Can you work these out from the model? Positions are in its coordinate system, mm. Round coordinates to 2 decimals unless told otherwise and drop trailing zeros. Write each loop counter-clockwise with the first axis right and the second up, starting at its lowest first coordinate (ties: lowest second). Pieces come first, ordered by that corner, then holes. Notation, with made-up numbers: M -19,19 L 37,19 A21 cw 37,40 Z; hole C 63.5,78.5 d3. An arc over 180 degrees is marked long. Use one line per item in the form item = value. Start each with the question number.
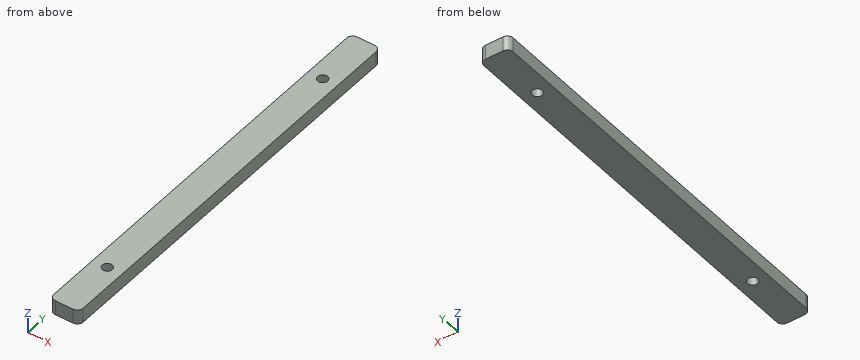
Autodesk Inventor part; units mm, degrees
ref_plane "YZ Plane" through (0, 0, 0) normal (1, 0, 0) x (0, 1, 0)
ref_plane "XZ Plane" through (0, 0, 0) normal (0, 1, 0) x (-1, 0, 0)
ref_plane "XY Plane" through (0, 0, 0) normal (0, 0, 1) x (1, 0, 0)
sketch "Sketch1" plane through (0, 0, 0) normal (0, 0, 1) x (1, 0, 0)
  line L0 (-5, -70) -> (5, -70)
  line L1 (5, -70) -> (5, 70)
  line L2 (5, 70) -> (-5, 70)
  line L3 (-5, 70) -> (-5, -70)
  line L4 (-5, -70) -> (5, 70) construction
  line L5 (5, -70) -> (-5, 70) construction
  point P0 (0, 0)
  dimension "d0" = 10
  dimension "d1" = 140
extrude "Extrusion1" add sketch "Sketch1" along normal blind 5
sketch "Sketch2" plane through (0, 0, 5) normal (0, 0, 1) x (1, 0, 0)
  line L0 (0, 50) -> (0, -50) construction
  point P0 (0, 0)
  point P1 (0, 0)
  dimension "d4" = 100
hole "Hole1" at (0, 50, 5) at (0, -50, 5) direction (0, 0, -1) diameter 3.4 depth 8 tip angle 118
fillet "Fillet1" radius 2 4 edges at (5, 70, 2.5) (-5, 70, 2.5) (5, -70, 2.5) (-5, -70, 2.5)
properties part number "ToslinkHalter" material "Polycarbonate, Clear"
1. If we section it at B-B (x = 0): List the corners of the cut face in (y, z) for me.
2. Will this pin go through, and if not, where does the flat tip stop? pin 1 (4 mm diameter, centred on x = 3.5, y = -12.5, fed in from -Z).
3. If we section it at A-A (y = -50): List the corners of the cut face in (x, z) for me, and give its area (3 significant figures).
4. Please list where these lines run through material, in increasing order: line 1 along Y through (x, z) = (0, 1.4); line 2 along X through (y, z) = (50, 3.45); line 3 along Y through (x, z) = (1, 0.3).
Model answer:
q1.outline = M -70,0 L -51.7,0 L -51.7,5 L -70,5 Z; M -48.3,0 L 48.3,0 L 48.3,5 L -48.3,5 Z; M 51.7,0 L 70,0 L 70,5 L 51.7,5 Z
q2.pin_1 = 0
q3.outline = M -5,0 L -1.7,0 L -1.7,5 L -5,5 Z; M 1.7,0 L 5,0 L 5,5 L 1.7,5 Z
q3.area = 33.0 mm2
q4.line_1 = -70 to -51.7, -48.3 to 48.3, 51.7 to 70
q4.line_2 = -5 to -1.7, 1.7 to 5
q4.line_3 = -70 to -51.37, -48.63 to 48.63, 51.37 to 70
